Work out the finished part from the listing and answer in its coordinate system (mm). Face numbers are marked on the shaded views. Coordinates: 2 decimals unless noted, no trailing zeros. Order: outer loops, then holes, each group sorted by start corner. A loop starts at its lowest first (then second) coordinate and runs counter-clockwise, first axis right, second up. Notation, with made-up numbers: M 2.5,87 L 16.5,87 A23 ccw 16.5,118 Z; hole C 4.5,81.5 d10. An arc over 180 degrees is marked long. Use a Markdown table: item, result.
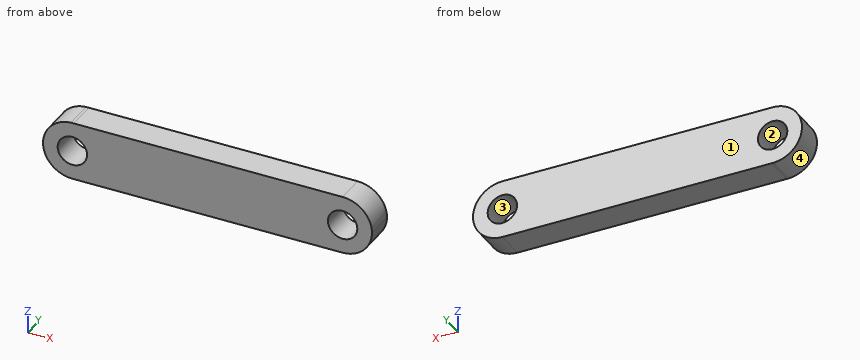
from build123d import *

# Parameters (mm, degrees)
F0_R     = 3.175
F1_DEPTH = 6.35


with BuildPart() as f1:
    # F0 (on Front) → F1 (new body)
    with BuildSketch(Plane.XZ):
        with BuildLine():
            Line((-55.794907, 6.912166), (-56.393981, 6.912093))
            ThreePointArc((-56.393981, 6.912093), (-62.443332, 0.503062), (-56.261799, -5.778576))
            Line((-56.261799, -5.778576), (-55.926036, -5.778589))
            ThreePointArc((-55.926036, -5.778589), (-51.544664, -3.861264), (-49.743676, 0.569198))
            ThreePointArc((-49.743676, 0.569198), (-51.499131, 4.952423), (-55.794907, 6.912166))
        make_face()
        with Locations((-56.093676, 0.569198)):
            Circle(F0_R, mode=Mode.SUBTRACT)
        with BuildLine():
            ThreePointArc((-55.794907, 6.912166), (-56.094445, 6.919198), (-56.393981, 6.912093))
            Line((-56.393981, 6.912093), (-55.794907, 6.912166))
        make_face()
        with BuildLine():
            Line((-55.926036, -5.778589), (-56.261799, -5.778576))
            ThreePointArc((-56.261799, -5.778576), (-56.093917, -5.780802), (-55.926036, -5.778589))
        make_face()
        with BuildLine():
            Line((2.325555, 6.919198), (-55.794907, 6.912166))
            ThreePointArc((-55.794907, 6.912166), (-51.499131, 4.952423), (-49.743676, 0.569198))
            ThreePointArc((-49.743676, 0.569198), (-51.544664, -3.861264), (-55.926036, -5.778589))
            Line((-55.926036, -5.778589), (2.326083, -5.780802))
            ThreePointArc((2.326083, -5.780802), (-4.023676, 0.568935), (2.325555, 6.919198))
        make_face()
        with BuildLine():
            ThreePointArc((8.676324, 0.569198), (6.81618, 5.059598), (2.325555, 6.919198))
            ThreePointArc((2.325555, 6.919198), (-4.023676, 0.568935), (2.326083, -5.780802))
            ThreePointArc((2.326083, -5.780802), (6.816367, -3.921015), (8.676324, 0.569198))
        make_face()
        with Locations((2.326324, 0.569198)):
            Circle(F0_R, mode=Mode.SUBTRACT)
    extrude(amount=F1_DEPTH)


solid = f1.part
1. Find the intervals of material crossed by probe 1 along X at (y, z) = (-5.5, -1); probe 2 along X at (y, z) = (-2, 3.25); probe 3 along Z at (x, y) = (-56, -1.5), in increasing order.
Answers below:
| item | result |
|---|---|
| probe 1 | -62.25 to -58.85, -53.33 to -0.43, 5.09 to 8.48 |
| probe 2 | -61.85 to -57.79, -54.39 to 0.63, 4.03 to 8.08 |
| probe 3 | -5.78 to -2.6, 3.74 to 6.92 |
2. Section D-D on z = 4.75 is taken. Determine the outline of the cut face in (x, y).
Answers below:
| item | result |
|---|---|
| outline | M -60.87,-6.35 L 7.11,-6.35 L 7.11,0 L -60.87,0 Z |
3. For a pull along Z with two mould halves and no side action, classify the marked faces 1, 2, 3 and 4 as +Z half, -Z half, draft (parallel to the pull), parting line (faces both ways), or undercut.
Answers below:
| item | result |
|---|---|
| face 1 | draft |
| face 2 | undercut |
| face 3 | undercut |
| face 4 | parting line |
4. Flat-ended cylindrical pins translate along their axes: P1, Ø5.5, axis at x = -56.09, z = 0.57, coming from the -Y side; P2, Ø1, axis at y = -5, z = -0.5, coming from the +X side; P3, Ø3, axis at x = -41.5, z = -4, coming from the +Y side; P4, Ø2, axis at x = -22.5, y = -4.5, coming from the +Z side. Find the tip coordinate at first contact, or state that the pin passes through.
Answers below:
| item | result |
|---|---|
| P1 | through |
| P2 | x = 8.65 |
| P3 | y = 0 |
| P4 | z = 6.92 |
5. Section A-A on y = -3.5 is taken. Determine the outline of the cut face in (x, z) (3 decimals).
Answers below:
| item | result |
|---|---|
| outline | M -56.394,6.912 A6.35 ccw -56.262,-5.779 A6.35 ccw -55.926,-5.779 L 2.326,-5.781 A6.35 ccw 2.326,6.919 L -55.795,6.912 A6.35 ccw Z; hole C -56.094,0.569 d6.35; hole C 2.326,0.569 d6.35 |
6. Section C-C on z = -0.5 is taken. Determine the outline of the cut face in (x, y).
Answers below:
| item | result |
|---|---|
| outline | M -62.35,-6.35 L -59.08,-6.35 L -59.08,0 L -62.35,0 Z; M -53.1,-6.35 L -0.66,-6.35 L -0.66,0 L -53.1,0 Z; M 5.32,-6.35 L 8.59,-6.35 L 8.59,0 L 5.32,0 Z |
7. Section B-B on x = 1 is taken. Determine the outline of the cut face in (y, z).
Answers below:
| item | result |
|---|---|
| outline | M -6.35,-5.78 L 0,-5.78 L 0,-2.32 L -6.35,-2.32 Z; M -6.35,3.45 L 0,3.45 L 0,6.92 L -6.35,6.92 Z |
